```python
from build123d import *

# Parameters (mm, degrees)
SKETCH1_W           = 40
SKETCH1_H           = 110.7
BOSS_EXTRUDE1_DEPTH = 10
SKETCH4_R           = 15
BOSS_EXTRUDE3_DEPTH = 10
SKETCH5_R           = 12.5
CUT_EXTRUDE2_DEPTH  = 8
SKETCH6_W           = 40
SKETCH6_H           = 10
CUT_EXTRUDE3_DEPTH  = 32.5
FILLET4_R           = 2.5
SKETCH11_R          = 1.5
SKETCH11_W          = 40
SKETCH11_H          = 10
BOSS_EXTRUDE4_DEPTH = 5


with BuildPart() as part:
    # Sketch1 → Boss-Extrude1 (new body)
    with BuildSketch(Plane.XY):
        Rectangle(SKETCH1_W, SKETCH1_H)
    extrude(amount=BOSS_EXTRUDE1_DEPTH)

    # Sketch4 → Boss-Extrude3 (add)
    with BuildSketch(Plane.XY.offset(10)):
        Circle(SKETCH4_R)
    extrude(amount=BOSS_EXTRUDE3_DEPTH)

    # Sketch5 → Cut-Extrude2 (cut)
    with BuildSketch(Plane.XY.offset(20)):
        Circle(SKETCH5_R)
    extrude(amount=-CUT_EXTRUDE2_DEPTH, mode=Mode.SUBTRACT)

    # Sketch6 → Cut-Extrude3 (cut)
    with BuildSketch(Plane(origin=(0, 55.35, 0), x_dir=(1, 0, 0), z_dir=(0, 1, 0))):
        with Locations((0, -5)):
            Rectangle(SKETCH6_W, SKETCH6_H)
    extrude(amount=-CUT_EXTRUDE3_DEPTH, mode=Mode.SUBTRACT)

    # Fillet4
    fillet4_edges = [part.edges().sort_by_distance(p)[0] for p in [
        (-20, 22.85, 5),
        (20, 22.85, 5),
    ]]
    fillet(fillet4_edges, radius=FILLET4_R)

    # Sketch11 → Boss-Extrude4 (add)
    with BuildSketch(Plane.XZ.offset(55.35)):
        with BuildLine():
            Line((-22.5, 15), (22.5, 15))
            ThreePointArc((22.5, 15), (26.035533906, 13.535533906), (27.5, 10))
            Line((27.5, 10), (27.5, 0))
            ThreePointArc((27.5, 0), (26.035533906, -3.535533906), (22.5, -5))
            Line((22.5, -5), (-22.5, -5))
            ThreePointArc((-22.5, -5), (-26.035533906, -3.535533906), (-27.5, 0))
            Line((-27.5, 0), (-27.5, 10))
            ThreePointArc((-27.5, 10), (-26.035533906, 13.535533906), (-22.5, 15))
        make_face()
        with Locations((-23.75, 5)):
            Circle(SKETCH11_R, mode=Mode.SUBTRACT)
        with Locations(Location((23.75, 5, 0), (0, 0, 180))):
            Circle(SKETCH11_R, mode=Mode.SUBTRACT)
        with Locations((0, 5)):
            Rectangle(SKETCH11_W, SKETCH11_H, mode=Mode.SUBTRACT)
    extrude(amount=-BOSS_EXTRUDE4_DEPTH)


solid = part.part
```
For this review, take the finished solid that the model builds, in its own axes (mm). A direction names the side the tool comes from. Round coordinates to 2 decimals unless told otherwise and drop trailing zeros. Write each loop counter-clockwise with the first axis right and the second up, starting at its lowest first coordinate (ties: lowest second). Pieces come first, ordered by that corner, then holes. Notation, with made-up numbers: (-4, -8) -> (51, -8) arc R17 ccw to (51, -4) -> close; hole circle Ø8 at (79.5, 27.5). An arc over 180 degrees is marked (long way). One line per question, with ' | ' between items. Start each with the question number.
1) Mouldability with a two-part tool opening along X and no side actions: class faces 1 (the flat face through (0, -21, 10)), 2 (the cylindrical face through (26.07, -52.89, -3.5)), 3 (the cylindrical face through (-25.25, -52.89, 5.07)) as +X half, -X half, draft (parallel to the pull), parting line (faces both ways), or undercut.
2) Wall thickness on line 1 along Y through (x, z) = (0, 17.25); line 2 along Y through (x, z) = (-8, 13.25); line 3 along X through (y, z) = (0.5, 12.75): over which ranges is each line inside the solid? List them lowest first.
3) Add section D-D (y = 0). Write out the cut boundary in (x, z).
4) For pin 1 Ø8 at (y, z) = (-11.5, 13) entering from +X; pin 2 Ø1 at (y, z) = (-4.5, 15.5) entering from -X; pin 3 Ø5 at (y, z) = (-9, 7) entering from -X, all flat-tipped, find the tip position at first contact; note any pin that passes through.
5) Add section C-C (z = 9). Write out the cut boundary in (x, y), and give its area (3 significant figures).
6) Add section B-B (x = 23.75). Write out the cut boundary in (y, z), and give its area (3 significant figures).
7) Add section A-A (z = 5). Write out the cut boundary in (x, y).
8) Machinability: for faces 4 (the flat face through (-20, -15, 5)), 5 (the flat face through (0, -13, 0)), 6 (the flat face through (20, -15, 5)), 7 (the cylindrical face through (-26.07, -52.89, 13.5)), 8 (the cylindrical face through (11.923, 3.755, 16.056)), which of the approach directions +Z, -Z, +X, -X, +Y, -Y give a long, thin tool a straight path to every point of the face, cutting with its end or side? Answer none if there is none.
Reported:
1) face 1: draft | face 2: +X half | face 3: undercut
2) line 1: y = -15 to -12.5, 12.5 to 15 | line 2: y = -55.35 to -50.35, -12.69 to -9.6, 9.6 to 12.69 | line 3: x = -14.99 to -12.49, 12.49 to 14.99
3) outline: (-20, 0) -> (20, 0) -> (20, 10) -> (15, 10) -> (15, 20) -> (12.5, 20) -> (12.5, 12) -> (-12.5, 12) -> (-12.5, 20) -> (-15, 20) -> (-15, 10) -> (-20, 10) -> close
4) pin 1: stops at x = 20 | pin 2: stops at x = -14.46 | pin 3: stops at x = -20
5) outline: (-27.5, -55.35) -> (27.5, -55.35) -> (27.5, -50.35) -> (20, -50.35) -> (20, 20.35) arc R2.5 ccw to (17.5, 22.85) -> (-17.5, 22.85) arc R2.5 ccw to (-20, 20.35) -> (-20, -50.35) -> (-27.5, -50.35) -> close | area: 3,200 mm²
6) outline: (-55.35, -4.84) -> (-50.35, -4.84) -> (-50.35, 3.5) -> (-55.35, 3.5) -> close; (-55.35, 6.5) -> (-50.35, 6.5) -> (-50.35, 14.84) -> (-55.35, 14.84) -> close | area: 83.4 mm²
7) outline: (-27.5, -55.35) -> (-25.25, -55.35) -> (-25.25, -50.35) -> (-27.5, -50.35) -> close; (-22.25, -55.35) -> (22.25, -55.35) -> (22.25, -50.35) -> (20, -50.35) -> (20, 20.35) arc R2.5 ccw to (17.5, 22.85) -> (-17.5, 22.85) arc R2.5 ccw to (-20, 20.35) -> (-20, -50.35) -> (-22.25, -50.35) -> close; (25.25, -55.35) -> (27.5, -55.35) -> (27.5, -50.35) -> (25.25, -50.35) -> close
8) face 4: +Z, -Z, -X, +Y | face 5: -Z, +X, -X, +Y | face 6: +Z, -Z, +X, +Y | face 7: +Z, -X, +Y, -Y | face 8: +Z
